CAD build for the part. Positions are in the model's coordinates, mm. A direction names the side the tool comes from. Coordinates: 2 decimals unless noted, no trailing zeros. Write each loop counter-clockwise with the first axis right and the second up, starting at its lowest first coordinate (ties: lowest second). Pieces come first, ordered by that corner, then holes. Notation, with made-up numbers: (19, 52) -> (33, 52) arc R17 ccw to (33, 74) -> close; hole circle Ø10 at (86.25, 35.5). An arc over 180 degrees is marked (long way). Answer as CSV lines item,"result".
```python
from build123d import *

# Parameters (mm, degrees)
F0_W      = 60
F0_H      = 49
F1_DEPTH  = 2.5
F1_FACE_W = 60
F1_FACE_H = 49
F2_DEPTH  = 3
F3_W      = 31.719639
F3_H      = 20.199234
F4_DEPTH  = 10


with BuildPart() as f1:
    # F0 (on Top) → F1 (new body)
    with BuildSketch(Plane.XY):
        with Locations((-18.378621, 19.452427)):
            Rectangle(F0_W, F0_H)
    extrude(amount=F1_DEPTH)

    # F1_face (on face) → F2 (join)
    with BuildSketch(Plane(origin=(-18.378621, 19.452427, 2.5), x_dir=(1, 0, 0), z_dir=(0, 0, 1))):
        Rectangle(F1_FACE_W, F1_FACE_H)
    extrude(amount=F2_DEPTH)

    # F3 (on face) → F4 (join)
    with BuildSketch(Plane.XY.offset(5.5)):
        with Locations((-14.857512, 18.312792)):
            Rectangle(F3_W, F3_H)
    extrude(amount=F4_DEPTH)


solid = f1.part
```
Item 1: Saw through at D-D on y = 2.5. Give the cut face in (x, z), and give its area (3 significant figures).
Answer below:
outline,"(-48.38, 0) -> (11.62, 0) -> (11.62, 5.5) -> (-48.38, 5.5) -> close"
area,"330 mm2"
Item 2: Saw through at C-C on z = 13.75. Give the cut face in (x, y), and give its area (3 significant figures).
Answer below:
outline,"(-30.72, 8.21) -> (1, 8.21) -> (1, 28.41) -> (-30.72, 28.41) -> close"
area,"641 mm2"
Item 3: Flat gauge pins, fed straight in: pin 1 (5 mm diameter, centred on y = 27, z = 9, fed in from +X); pin 2 (5 mm diameter, centred on x = -11, z = 12, fed in from +Y); pin 3 (8 mm diameter, centred on x = -9.5, z = 12.5, fed in from -Y). Where does each tip first touch, or does it go through?
Answer below:
pin 1,"stops at x = 1"
pin 2,"stops at y = 28.41"
pin 3,"stops at y = 8.21"
Item 4: Saw through at B-B on y = 13. Give the cut face in (x, z), and give its area (3 significant figures).
Answer below:
outline,"(-48.38, 0) -> (11.62, 0) -> (11.62, 5.5) -> (1, 5.5) -> (1, 15.5) -> (-30.72, 15.5) -> (-30.72, 5.5) -> (-48.38, 5.5) -> close"
area,"647 mm2"
Item 5: 3-axis set-ups, long thin cutter, end or side, ignore diameter. For faces 1 (the flat face through (-30.717, 18, 10)), 2 (the flat face through (-15, 8.213, 10)), 3 (the flat face through (-15, 28.412, 10)), 4 (the flat face through (1.002, 18, 10)): which of +Z, -Z, +X, -X, +Y, -Y reach the whole face in a straight line?
Answer below:
face 1,"+Z, -X, +Y, -Y"
face 2,"+Z, +X, -X, -Y"
face 3,"+Z, +X, -X, +Y"
face 4,"+Z, +X, +Y, -Y"
Item 6: Wall check: line 1 (Y direction, x = -14, z = 9.75); line 2 (X direction, y = 17.5, z = 15.25); line 3 (Z direction, x = -44, y = 36). Give the ranges that are in metal, low to high. Write a range as from..to.
Answer below:
line 1,"y = 8.21..28.41"
line 2,"x = -30.72..1"
line 3,"z = 0..5.5"
Item 7: Saw through at A-A on x = -2. Give the cut face in (y, z).
Answer below:
outline,"(-5.05, 0) -> (43.95, 0) -> (43.95, 5.5) -> (28.41, 5.5) -> (28.41, 15.5) -> (8.21, 15.5) -> (8.21, 5.5) -> (-5.05, 5.5) -> close"
